Read the model definition and answer for the solid it produces. Units are mm, in the model's axes. Face numbers are marked on the shaded views. A direction names the side the tool comes from. Coordinates: 2 decimals unless noted, no trailing zeros. Write each loop counter-clockwise with the first axis right and the second up, starting at its lowest first coordinate (ties: lowest second). Pieces come first, ordered by that corner, then holes.
(1) Given pin 1 (6 mm diameter, centred on x = 20.5, y = 10, fed in from -Z); pin 2 (1.5 mm diameter, centred on y = 13.5, z = 10, fed in from -X); pin 3 (10 mm diameter, centred on x = 6, z = 15, fed in from -Y); pin 4 (2 mm diameter, centred on y = 17, z = 12, fed in from -X), each flat-ended and moving along its own axis, determine where each tip first touches the part or whether it passes through.
(2) The part is cut by section A-A, the plane y = 2.5. Determine the outline of the cut face in (x, z).
(3) The part is cut by section C-C, the plane z = 10. Determine the outline of the cut face in (x, y), and give its area (3 significant figures).
(4) Which of the six approach directions +Z, -Z, +X, -X, +Y, -Y give full straight-line access (tool end or side, diameter ignored) to the marked faces 4 and 5?
(5) Determine the mould class of the marked faces 1, 2 and 3 for opening direction Y: pulls with the +Y half, pulls with the -Y half, needs draft (parallel to the pull), parting line crosses it, or undercut.
(6) The part is cut by section D-D, the plane z = 6. Determine the outline of the cut face in (x, y), and give its area (4 significant figures).
(7) Straight lines are drawn through the part: line 1 along Z through (x, y) = (15, 21.6); line 2 along Y through (x, z) = (24.95, 10); line 3 along Y through (x, z) = (17, 11). For each, find the intervals that lie inside material, in ascending order.
(8) The part is cut by section B-B, the plane x = 15. Determine the outline of the cut face in (y, z).
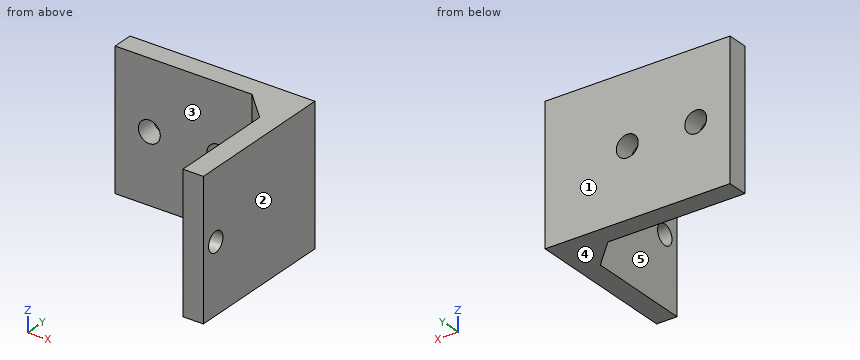
Autodesk Inventor part; units mm, degrees
ref_plane "YZ Plane" through (0, 0, 0) normal (1, 0, 0) x (0, 1, 0)
ref_plane "XZ Plane" through (0, 0, 0) normal (0, 1, 0) x (-1, 0, 0)
ref_plane "XY Plane" through (0, 0, 0) normal (0, 0, 1) x (1, 0, 0)
sketch "Sketch1" plane through (0, 0, 0) normal (0, 0, 1) x (1, 0, 0)
  line L0 (0, 22.5) -> (27, 22.5)
  line L1 (27, 22.5) -> (27, 0)
  line L2 (27, 0) -> (24, 0)
  line L3 (24, 0) -> (24, 19.5)
  line L4 (24, 19.5) -> (0, 19.5)
  line L5 (0, 19.5) -> (0, 22.5)
  line L6 (-5.4, 0) -> (32.4, 0) construction
  line L7 (0, -4.5) -> (0, 27) construction
  point P0 (0, 0)
  dimension "d0" = 3
  dimension "d1" = 3
  dimension "d2" = 22.5
  dimension "d3" = 27
extrude "Extrusion1" add sketch "Sketch1" along normal blind 20
chamfer "Chamfer1" distance 4 angle 45 1 edges at (24, 19.5, 10)
sketch "Sketch2" plane through (27, 0, 0) normal (1, 0, 0) x (0, 0, -1)
  circle A0 centre (-10, 2.5) radius 1.45
  line L0 (0, 0) -> (-20, 0) construction
  line L1 (-10, 0) -> (-10, 2.5) construction
  dimension "d9" = 2.9
  dimension "d10" = 2.5
extrude "Extrusion2" cut sketch "Sketch2" against normal up to surface (3 mm away)
sketch "Sketch3" plane through (0, 19.5, 0) normal (0, -1, 0) x (1, 0, 0)
  circle A0 centre (5, 10) radius 1.6
  circle A1 centre (15, 10) radius 1.6
  line L0 (0, 0) -> (0, 20) construction
  line L1 (0, 10) -> (20, 10) construction
  line L2 (20, 20) -> (20, 0) construction
  dimension "d13" = 3.2
  dimension "d14" = 5
  dimension "d15" = 5
extrude "Extrusion3" cut sketch "Sketch3" against normal up to surface (3 mm away)
properties part number "Motor_Holder"
Computed:
1. pin 1: passes through
1. pin 2: stops at x = 24
1. pin 3: stops at y = 19.5
1. pin 4: stops at x = 21.5
2. outline: (24, 0) - (27, 0) - (27, 8.55) - (24, 8.55) - close; (24, 11.45) - (27, 11.45) - (27, 20) - (24, 20) - close
3. outline: (0, 19.5) - (3.4, 19.5) - (3.4, 22.5) - (0, 22.5) - close; (6.6, 19.5) - (13.4, 19.5) - (13.4, 22.5) - (6.6, 22.5) - close; (16.6, 19.5) - (20, 19.5) - (24, 15.5) - (24, 3.95) - (27, 3.95) - (27, 22.5) - (16.6, 22.5) - close; (24, 0) - (27, 0) - (27, 1.05) - (24, 1.05) - close
3. area: 120 mm2
4. face 4: -Z, +X, -X, +Y, -Y
4. face 5: +Z, -Z, -X, -Y
5. face 1: pulls with the +Y half
5. face 2: needs draft
5. face 3: pulls with the -Y half
6. outline: (0, 19.5) - (20, 19.5) - (24, 15.5) - (24, 0) - (27, 0) - (27, 22.5) - (0, 22.5) - close
6. area: 147.5 mm2
7. line 1: z = 0 to 8.4, 11.6 to 20
7. line 2: y = 0 to 1.05, 3.95 to 22.5
7. line 3: y = 19.5 to 22.5
8. outline: (19.5, 0) - (22.5, 0) - (22.5, 8.4) - (19.5, 8.4) - close; (19.5, 11.6) - (22.5, 11.6) - (22.5, 20) - (19.5, 20) - close
